from build123d import *

# Parameters (mm, degrees)
SKICA1_W                    = 50
SKICA1_H                    = 60
P_IDAT_VYSUNUT_M2_DEPTH     = 3
SKICA3_W                    = 64
SKICA3_H                    = 74
SKICA3_W_2                  = 50
SKICA3_H_2                  = 60
VYSUNOUT_TENKOST_NN_1_DEPTH = 35
SKICA4_W                    = 66
SKICA4_H                    = 100
SKICA4_R                    = 2.15
SKICA4_W_2                  = 50
SKICA4_H_2                  = 60
P_IDAT_VYSUNUT_M5_DEPTH     = 3
SKICA2_R                    = 6
SKICA2_R_2                  = 2
VYSUNOUT_TENKOST_NN_2_DEPTH = 3
ZAOBLIT2_R                  = 3
ODEBRAT_VYSUNUT_M3_REACH    = 107.868
SKICA9_R                    = 7
ZAOBLIT4_R                  = 3
ZAOBLIT5_R                  = 3
ZAOBLIT6_R                  = 3
ZAOBLIT7_R                  = 3
SKICA10_R                   = 1.75
ODEBRAT_VYSUNUT_M4_DEPTH    = 30


with BuildPart() as part:
    # Skica1 → P_idat vysunut_m2 (new body)
    with BuildSketch(Plane.XY):
        with Locations((25, 30)):
            Rectangle(SKICA1_W, SKICA1_H)
    extrude(amount=P_IDAT_VYSUNUT_M2_DEPTH)



with BuildPart() as body_2:
    # Skica3 → Vysunout tenkost_nn_1 (new body)
    with BuildSketch(Plane.XY.offset(3)):
        with Locations((25, 30)):
            Rectangle(SKICA3_W, SKICA3_H)
        with Locations((25, 30)):
            Rectangle(SKICA3_W_2, SKICA3_H_2, mode=Mode.SUBTRACT)
    extrude(amount=VYSUNOUT_TENKOST_NN_1_DEPTH)


with BuildPart() as part_1:
    add(part.part)

    add(body_2.part)  # P_idat vysunut_m5 merges body 2
    # Skica4 → P_idat vysunut_m5 (add)
    with BuildSketch(Plane(origin=(0, 0, 0), x_dir=(-1, 0, 0), z_dir=(0, 0, -1))):
        with Locations((-25, 30)):
            Rectangle(SKICA4_W, SKICA4_H)
        with Locations((-53, 75)):
            Circle(SKICA4_R, mode=Mode.SUBTRACT)
        with Locations((3, 75)):
            Circle(SKICA4_R, mode=Mode.SUBTRACT)
        with Locations((3, -15)):
            Circle(SKICA4_R, mode=Mode.SUBTRACT)
        with Locations((-53, -15)):
            Circle(SKICA4_R, mode=Mode.SUBTRACT)
        with Locations((-25, 30)):
            Rectangle(SKICA4_W_2, SKICA4_H_2, mode=Mode.SUBTRACT)
    extrude(amount=-P_IDAT_VYSUNUT_M5_DEPTH)

    # Skica2 → Vysunout tenkost_nn_2 (add)
    # profile 1 of 4: a face of its own
    with BuildSketch(Plane.XY.offset(3)):
        with Locations((9, 53)):
            Circle(SKICA2_R)
        with Locations((9, 53)):
            Circle(SKICA2_R_2, mode=Mode.SUBTRACT)
    # profile 2 of 4: a face of its own
    with BuildSketch(Plane.XY.offset(3)):
        with Locations((35, 53)):
            Circle(SKICA2_R)
        with Locations((35, 53)):
            Circle(SKICA2_R_2, mode=Mode.SUBTRACT)
    # profile 3 of 4: a face of its own
    with BuildSketch(Plane.XY.offset(3)):
        with Locations((35, 8)):
            Circle(SKICA2_R)
        with Locations((35, 8)):
            Circle(SKICA2_R_2, mode=Mode.SUBTRACT)
    # profile 4 of 4: a face of its own
    with BuildSketch(Plane.XY.offset(3)):
        with Locations((9, 8)):
            Circle(SKICA2_R)
        with Locations((9, 8)):
            Circle(SKICA2_R_2, mode=Mode.SUBTRACT)
    extrude(amount=VYSUNOUT_TENKOST_NN_2_DEPTH)

    # Zaoblit2
    zaoblit2_edges = [part_1.edges().sort_by_distance(p)[0] for p in [
        (-7, 67, 20.5),
        (-7, -7, 20.5),
        (57, -7, 20.5),
        (57, 67, 20.5),
    ]]
    fillet(zaoblit2_edges, radius=ZAOBLIT2_R)

    # Skica9 → Odebrat vysunut_m3 (cut, up to next)
    with BuildSketch(Plane(origin=(0, 0, 0), x_dir=(0, 0, -1), z_dir=(1, 0, 0)), mode=Mode.PRIVATE) as odebrat_vysunut_m3_sk1:
        with Locations((-28.5, 20)):
            Circle(SKICA9_R)
    odebrat_vysunut_m3_tool1 = extrude(odebrat_vysunut_m3_sk1.sketch, amount=-ODEBRAT_VYSUNUT_M3_REACH, mode=Mode.PRIVATE) & part_1.part
    add(odebrat_vysunut_m3_tool1.solids().sort_by_distance((0, 20, 28.5))[0], mode=Mode.SUBTRACT)

    # Zaoblit4
    zaoblit4_edges = [part_1.edges().sort_by_distance(p)[0] for p in [
        (50, 60, 20.5),
    ]]
    fillet(zaoblit4_edges, radius=ZAOBLIT4_R)

    # Zaoblit5
    zaoblit5_edges = [part_1.edges().sort_by_distance(p)[0] for p in [
        (50, 0, 20.5),
    ]]
    fillet(zaoblit5_edges, radius=ZAOBLIT5_R)

    # Zaoblit6
    zaoblit6_edges = [part_1.edges().sort_by_distance(p)[0] for p in [
        (0, 0, 20.5),
    ]]
    fillet(zaoblit6_edges, radius=ZAOBLIT6_R)

    # Zaoblit7
    zaoblit7_edges = [part_1.edges().sort_by_distance(p)[0] for p in [
        (0, 60, 20.5),
    ]]
    fillet(zaoblit7_edges, radius=ZAOBLIT7_R)

    # Skica10 → Odebrat vysunut_m4 (cut)
    with BuildSketch(Plane.XY.offset(38)):
        with Locations((-2.5, 62.5)):
            Circle(SKICA10_R)
        with Locations((52.5, 62.5)):
            Circle(SKICA10_R)
        with Locations((52.5, -2.5)):
            Circle(SKICA10_R)
        with Locations((-2.5, -2.5)):
            Circle(SKICA10_R)
    extrude(amount=-ODEBRAT_VYSUNUT_M4_DEPTH, mode=Mode.SUBTRACT)


solid = part_1.part
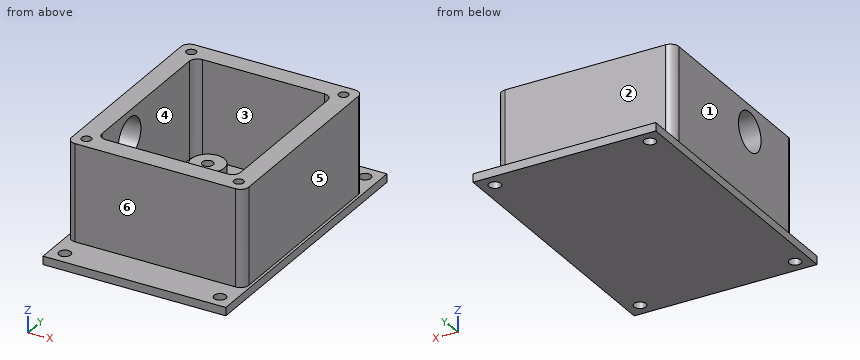
Check sheet for the modelled part. Datum: model origin and axes. Units: mm. Face numbers are marked on the shaded views. A direction names the side the tool comes from. Round coordinates to 2 decimals unless told otherwise and drop trailing zeros. Loops run counter-clockwise (first coordinate to the right, second up) from the corner with the lowest first, then second, coordinate; pieces in that order, holes last.
1. Gauge pin test, flat ends, axial feed: pin 1 Ø3 at (x, y) = (46.5, 37.5) entering from +Z; pin 2 Ø1.5 at (y, z) = (8, 4) entering from -X; pin 3 Ø2 at (x, y) = (10, 52) entering from +Z; pin 4 Ø4 at (x, y) = (-3, 75) entering from -Z. Record the tip position at first contact, or that the pin passes through.
2. Sectioned sample at C-C on z = 9.5. Record the boundary of the cut face in (x, y), and give its area (3 significant figures).
3. Set-up check for the marked faces 1, 2 and 3: record each of +Z, -Z, +X, -X, +Y, -Y from which the full face is reachable in a straight line by a thin tool's end or side.
4. Sectioned sample at B-B on x = -2. Record the boundary of the cut face in (y, z).
5. Mould release check, pull along X, two halves, no side actions. Record for the marked faces 4, 5 and 6: released by +X, released by -X, zero draft, split by the parting line, or undercut.
6. Sectioned sample at D-D on y = 75. Record the boundary of the cut face in (x, z), and give its area (3 significant figures).
7. Sectioned sample at A-A on y = 20. Record the boundary of the cut face in (x, z), and give its area (3 significant figures).
8. Scan lines: probe 1 along Y at (x, z) = (52.5, 30.75); probe 2 along Y at (x, z) = (3, 36.5); probe 3 along X at (y, z) = (9, 25.5). Record each from-to range of solid material in increasing order.
Recorded:
1. pin 1: stops at z = 3
1. pin 2: stops at x = -7
1. pin 3: stops at z = 6
1. pin 4: passes through
2. outline: (-7, -4) arc R3 ccw to (-4, -7) - (54, -7) arc R3 ccw to (57, -4) - (57, 64) arc R3 ccw to (54, 67) - (-4, 67) arc R3 ccw to (-7, 64) - close; hole circle Ø3.5 at (-2.5, -2.5); hole circle Ø3.5 at (-2.5, 62.5); hole (0, 3) arc R3 ccw to (3, 0) - (47, 0) arc R3 ccw to (50, 3) - (50, 57) arc R3 ccw to (47, 60) - (3, 60) arc R3 ccw to (0, 57) - close; hole circle Ø3.5 at (52.5, -2.5); hole circle Ø3.5 at (52.5, 62.5)
2. area: 1,700 mm2
3. face 1: +Z, -X, +Y, -Y
3. face 2: +Z, +X, -X, +Y
3. face 3: +Z
4. outline: (-20, 0) - (-16.9, 0) - (-16.9, 3) - (-20, 3) - close; (-13.1, 0) - (73.1, 0) - (73.1, 3) - (67, 3) - (67, 38) - (64.18, 38) - (64.18, 8) - (60.82, 8) - (60.82, 38) - (-0.82, 38) - (-0.82, 8) - (-4.18, 8) - (-4.18, 38) - (-7, 38) - (-7, 3) - (-13.1, 3) - close; (76.9, 0) - (80, 0) - (80, 3) - (76.9, 3) - close; hole circle Ø14 at (20, 28.5)
5. face 4: undercut
5. face 5: released by +X
5. face 6: zero draft
6. outline: (-8, 0) - (-5.15, 0) - (-5.15, 3) - (-8, 3) - close; (-0.85, 0) - (50.85, 0) - (50.85, 3) - (-0.85, 3) - close; (55.15, 0) - (58, 0) - (58, 3) - (55.15, 3) - close
6. area: 172 mm2
7. outline: (-8, 0) - (58, 0) - (58, 3) - (57, 3) - (57, 38) - (50, 38) - (50, 3) - (0, 3) - (0, 21.5) - (-7, 21.5) - (-7, 3) - (-8, 3) - close; (-7, 35.5) - (0, 35.5) - (0, 38) - (-7, 38) - close
7. area: 590 mm2
8. probe 1: y = -7 to -4.25, -0.75 to 60.75, 64.25 to 67
8. probe 2: y = -7 to 0, 60 to 67
8. probe 3: x = -7 to 0, 50 to 57
